Check sheet for the modelled part. Datum: model origin and axes. Units: mm. A direction names the side the tool comes from. Round coordinates to 2 decimals unless told otherwise and drop trailing zeros. Order: outer loops, then holes, each group sorted by start corner. A loop starts at its lowest first (then second) coordinate and runs counter-clockwise, first axis right, second up.
(1) Depth check by flat-ended pin: pin 1 (14.5 mm diameter, centred on x = 0, y = 0, fed in from +Z); pin 2 (5 mm diameter, centred on y = -4.5, z = 0, fed in from +X); pin 3 (6 mm diameter, centred on x = -1, z = -0.5, fed in from -Y); pin 4 (5 mm diameter, centred on x = -13.5, z = 4, fed in from -Y). Enter the tip coordinate at first touch or a pass-through.
(2) Thickness scan on probe 1 along Y at (x, z) = (0, -3.5); probe 2 along Z at (x, y) = (11, -13); probe 3 along Z at (x, y) = (15.5, 11) (3 decimals). Record the ranges inside material, lowest first.
(3) Mould release check, pull along X, two halves, no side actions. Record for faces 1 (the cylindrical face through (-1.38, -6.2, -0.08)), 2 (the cylindrical face through (18.17, 5.72, -4.74)), 3 (the flat face through (6, 17, 3.175)): released by +X, released by -X, zero draft, split by the parting line, or undercut.
(4) Sectioned sample at C-C, the plane z = -4.75. Enter the section's corners in (x, y).
(5) Sectioned sample at D-D, the plane z = 1.5. Enter the section's corners in (x, y), and give its area (3 significant figures).
(6) Tool access check on faces 4 (the flat face through (8, 0, 6.35)), 5 (the flat face through (6, -17, -3.175)). Record the directions out of +Z, -Z, +X, -X, +Y, -Y that give a thin tool (end or side, any length) a straight path to the whole face; none if there is none.
```python
from build123d import *

# Parameters (mm, degrees)
SKETCH1_R      = 19.05
SKETCH1_R_2    = 6.35
EXTRUDE1_DEPTH = 6.35
CHAMFER1_SIZE  = 0.79375


with BuildPart() as part:
    # Sketch1 → Extrude1 (new, symmetric)
    with BuildSketch(Plane.XY):
        Circle(SKETCH1_R)
        Circle(SKETCH1_R_2, mode=Mode.SUBTRACT)
    extrude(amount=EXTRUDE1_DEPTH, both=True)

    # Chamfer1
    chamfer1_edges = [part.edges().sort_by_distance(p)[0] for p in [
        (-6.35, 0, -6.35),
        (-6.35, 0, 6.35),
    ]]
    chamfer(chamfer1_edges, length=CHAMFER1_SIZE)

    # Sketch2 → Cut-Revolve1 (revolve, cut)
    with BuildSketch(Plane(origin=(0, 0, 0), x_dir=(0, 0, -1), z_dir=(1, 0, 0)), mode=Mode.PRIVATE) as cut_revolve1_sk:
        with BuildLine():
            Line((-3.175, 17.4625), (-3.175, 19.05))
            Line((-3.175, 19.05), (3.175, 19.05))
            Line((3.175, 19.05), (3.175, 17.4625))
            ThreePointArc((3.175, 17.4625), (0, 14.2875), (-3.175, 17.4625))
        make_face()
    revolve(cut_revolve1_sk.sketch.rotate(Axis((0, 0, 6.35), (0, 0, -1)), 180), axis=Axis((0, 0, 6.35), (0, 0, -1)), mode=Mode.SUBTRACT)


solid = part.part
```
Derived:
1. pin 1: stops at z = 6.35
1. pin 2: stops at x = 14.92
1. pin 3: stops at y = -19.05
1. pin 4: stops at y = -15.55
2. probe 1: y = -19.05 to -6.35, 6.35 to 19.05
2. probe 2: z = -6.35 to -3.15, 3.15 to 6.35
2. probe 3: z = -6.35 to -3.175, 3.175 to 6.35
3. face 1: undercut
3. face 2: split by the parting line
3. face 3: zero draft
4. outline: circle Ø38.1 at (0, 0); hole circle Ø12.7 at (0, 0)
5. outline: circle Ø29.33 at (0, 0); hole circle Ø12.7 at (0, 0)
5. area: 549 mm2
6. face 4: +Z, +X, -X, +Y, -Y
6. face 5: none
